Geometry check sheet. Reference: drawing and pictorial views, mm from the part's lowest x, y, z. Give positions to 0.01 mm unless a question says otherwise; leave off trailing zeros. Order: outer loops, then holes, each group sorted by start corner. A loop starts at its lowest first (then second) coordinate and runs counter-clockwise, first axis right, second up. Notation, with made-up numbers: M 87.5,-34.75 L 103.5,-34.75 A15 ccw 103.5,-5.75 Z; hole C 73.5,-11 d9. An arc over 180 degrees is marked long. Use CSV: the item, a comma, the result in double quotes. Start each with the question number.
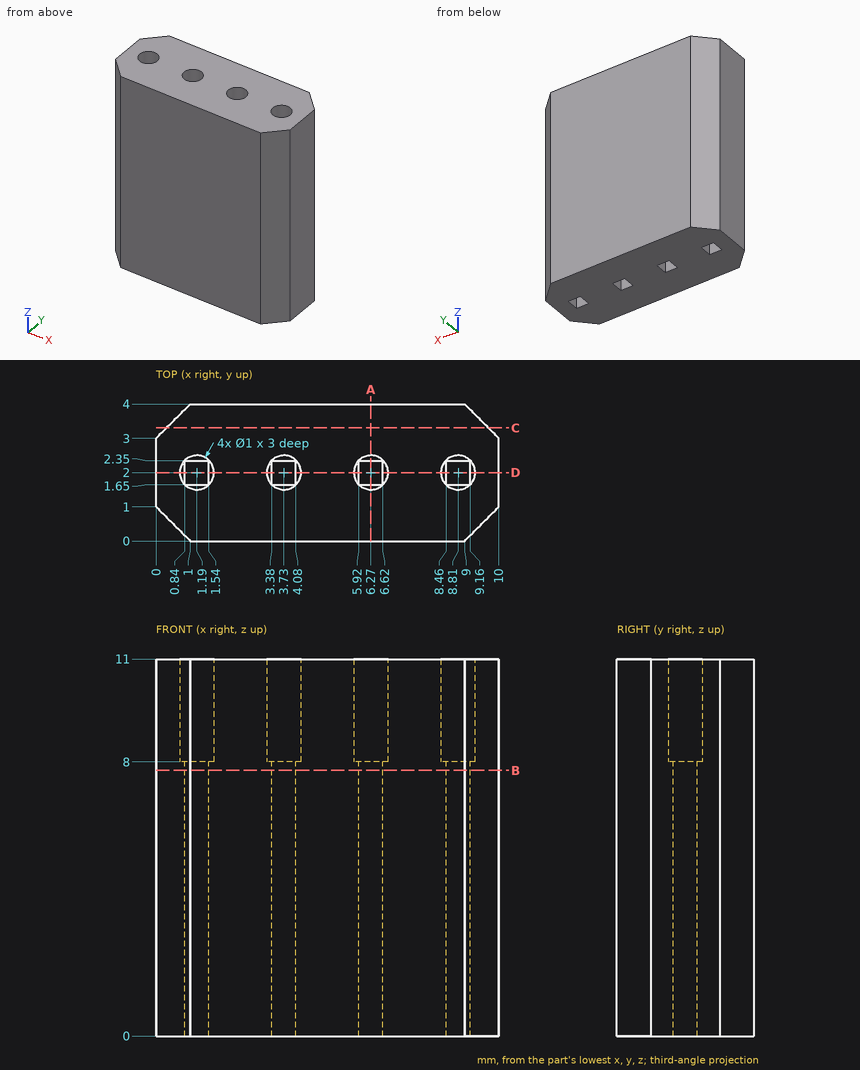
(1) Sectioned sample at A-A on x = 6.27. Record the cut outline in (y, z), then the cut area to 3 significant figures.
(2) Sectioned sample at D-D on y = 2. Give the number of separate pieces and of enclosed holes in the cut face, then the cut area to 3 significant figures.
(3) Sectioned sample at B-B on z = 7.75. Record the cut outline in (x, y), then the cut area to 3 significant figures.
(4) Thickness scan on line 1 (Y direction, x = 6.27, z = 10.35); line 2 (Y direction, x = 6.5, z = 9.75); line 3 (Z direction, x = 3.75, y = 2.4). Record the ranges inside material, lowest first.
(5) Sectioned sample at C-C on y = 3.3. Record the cut outline in (x, z).
Responses:
1,outline,"M 0,0 L 1.65,0 L 1.65,8 L 1.5,8 L 1.5,11 L 0,11 Z; M 2.35,0 L 4,0 L 4,11 L 2.5,11 L 2.5,8 L 2.35,8 Z"
1,area,"35.4 mm2"
2,separate pieces,"5"
2,enclosed holes,"0"
2,area,"75.6 mm2"
3,outline,"M 0,1 L 1,0 L 9,0 L 10,1 L 10,3 L 9,4 L 1,4 L 0,3 Z; hole M 0.84,1.65 L 1.54,1.65 L 1.54,2.35 L 0.84,2.35 Z; hole M 3.38,1.65 L 4.08,1.65 L 4.08,2.35 L 3.38,2.35 Z; hole M 5.92,1.65 L 6.62,1.65 L 6.62,2.35 L 5.92,2.35 Z; hole M 8.46,1.65 L 9.16,1.65 L 9.16,2.35 L 8.46,2.35 Z"
3,area,"36.0 mm2"
4,line 1,"0 to 1.5, 2.5 to 4"
4,line 2,"0 to 1.56, 2.44 to 4"
4,line 3,"0 to 8"
5,outline,"M 0.3,0 L 9.7,0 L 9.7,11 L 0.3,11 Z"
